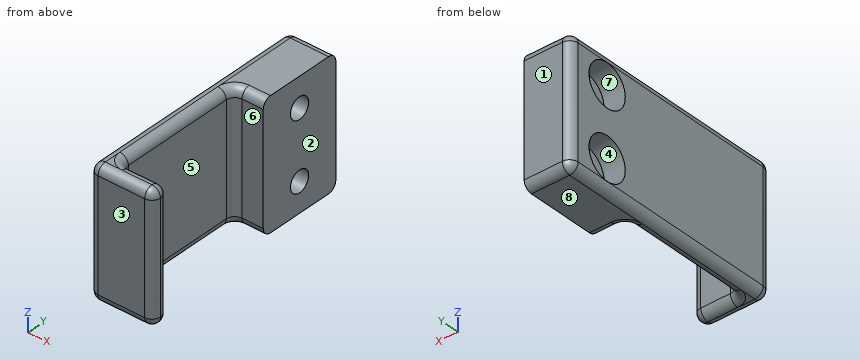
```python
from build123d import *

# Parameters (mm, degrees)
EXTRUDE_1_DEPTH     = 30
SKETCH_3_W          = 7
SKETCH_3_H          = 20
EXTRUDE_2_DEPTH     = 30
SKETCH_2_R          = 2.5
CUT_EXTRUDE_1_DEPTH = 30
FILLET_1_R          = 2
FILLET_2_R          = 2
FILLET_3_R          = 2
FILLET_5_R          = 2
SKETCH_4_R          = 5
CUT_EXTRUDE_2_DEPTH = 5


with BuildPart() as part:
    # 스케치1 → 보스-돌출1 (new body)
    with BuildSketch(Plane.XY):
        Polygon((-41.818181818, 31.136363636), (-37.818181818, 31.136363636), (-37.818181818, -19.863636364), (-26.818181818, -19.863636364), (-26.818181818, -23.863636364), (-32.727272727, -23.863636364), (-41.818181818, -23.863636364), align=None)
    extrude(amount=EXTRUDE_1_DEPTH)

    # 스케치3 → 보스-돌출2 (add)
    with BuildSketch(Plane.XY.offset(30)):
        with Locations((-34.318181818, 21.136363636)):
            Rectangle(SKETCH_3_W, SKETCH_3_H)
    extrude(amount=-EXTRUDE_2_DEPTH)

    # 스케치2 → 컷-돌출1 (cut)
    with BuildSketch(Plane.ZY.offset(41.818181818)):
        with Locations((7, 21.136363636)):
            Circle(SKETCH_2_R)
        with Locations((23, 21.136363636)):
            Circle(SKETCH_2_R)
    extrude(amount=-CUT_EXTRUDE_1_DEPTH, mode=Mode.SUBTRACT)

    # 필렛1
    fillet_1_edges = [part.edges().sort_by_distance(p)[0] for p in [
        (-37.818181818, -19.863636364, 15),
        (-37.818181818, 11.136363636, 15),
    ]]
    fillet(fillet_1_edges, radius=FILLET_1_R)

    # 필렛2
    fillet_2_edges = [part.edges().sort_by_distance(p)[0] for p in [
        (-41.818181818, -23.863636364, 15),
    ]]
    fillet(fillet_2_edges, radius=FILLET_2_R)

    # 필렛3
    fillet_3_edges = [part.edges().sort_by_distance(p)[0] for p in [
        (-26.818181818, -23.863636364, 15),
        (-26.818181818, -19.863636364, 15),
        (-41.818181818, 31.136363636, 15),
    ]]
    fillet(fillet_3_edges, radius=FILLET_3_R - 0.0001)  # a hair under: the kernel refuses the full size

    # 필렛5
    fillet_5_edges = [part.edges().sort_by_distance(p)[0] for p in [
        (-35.318231818, 31.136363636, 30),
        (-33.318181818, 11.136363636, 0),
        (-37.818181818, -4.363636364, 0),
        (-37.818181818, -4.363636364, 30),
        (-33.318181818, 11.136363636, 30),
        (-37.232395381, 10.550577199, 30),
        (-37.232395381, 10.550577199, 0),
        (-37.232395381, -19.277849926, 0),
        (-37.232395381, -19.277849926, 30),
        (-34.318131818, -23.863636364, 0),
        (-34.318131818, -23.863636364, 30),
        (-41.232395381, -23.277849926, 0),
        (-41.232395381, -23.277849926, 30),
        (-41.818181818, 3.636413636, 0),
        (-32.318131818, -19.863636364, 0),
        (-41.23242467, 30.550606488, 0),
        (-27.403938966, -20.449393512, 0),
        (-27.403938966, -23.277879215, 0),
        (-41.818181818, 3.636413636, 30),
        (-35.318231818, 31.136363636, 0),
        (-32.318131818, -19.863636364, 30),
        (-41.23242467, 30.550606488, 30),
        (-27.403938966, -20.449393512, 30),
        (-27.403938966, -23.277879215, 30),
    ]]
    fillet(fillet_5_edges, radius=FILLET_5_R - 0.0001)  # a hair under: the kernel refuses the full size

    # 스케치4 → 컷-돌출2 (cut)
    with BuildSketch(Plane.ZY.offset(41.818181818)):
        with Locations((7, 21.136363636)):
            Circle(SKETCH_4_R)
        with Locations((23, 21.136363636)):
            Circle(SKETCH_4_R)
    extrude(amount=-CUT_EXTRUDE_2_DEPTH, mode=Mode.SUBTRACT)


solid = part.part
```
Geometry check sheet. Reference: the model listing, model coordinates, mm. Face numbers are marked on the shaded views. A direction names the side the tool comes from. Coordinates: 2 decimals unless noted, no trailing zeros.
Item 1: Section check B-B (x = -34). Count the separate pieces of the cut face and the enclosed holes in it, plus the area to 3 significant figures.
Item 2: Scan lines: line 1 along Y through (x, z) = (-34.9, 23); line 2 along Y through (x, z) = (-33, 22.25); line 3 along Y through (x, z) = (-35.75, 27.5). Record each from-to range of solid material in increasing order.
Item 3: Tool access check on the marked faces 1, 2, 3, 4 and 5. Record the directions out of +Z, -Z, +X, -X, +Y, -Y that give a thin tool (end or side, any length) a straight path to the whole face; none if there is none.
Item 4: Depth check by flat-ended pin: pin 1 (5 mm diameter, centred on y = 23, z = 5.5, fed in from -X); pin 2 (8 mm diameter, centred on y = -7.5, z = 12, fed in from +X); pin 3 (9 mm diameter, centred on y = 21.14, z = 23, fed in from +X); pin 4 (4.5 mm diameter, centred on y = 21.14, z = 7, fed in from -X). Enter the tip coordinate at first touch or a pass-through.
Item 5: Mould release check, pull along Z, two halves, no side actions. Record for the marked faces 6, 7 and 8: released by +Z, released by -Z, zero draft, split by the parting line, or undercut.
Check sheet entries:
1. separate pieces: 2
1. enclosed holes: 2
1. area: 674 mm2
2. line 1: y = -23.86 to -19.86, 11.14 to 18.64, 23.64 to 31.14
2. line 2: y = -23.86 to -19.86, 11.14 to 18.75, 23.52 to 31.14
2. line 3: y = -23.86 to -19.86, 11.14 to 31.14
3. face 1: +Z, -Z, +X, -X, +Y
3. face 2: +Z, -Z, +X, +Y
3. face 3: +Z, -Z, +X, -X, -Y
3. face 4: -X
3. face 5: +Z, -Z, +X
4. pin 1: stops at x = -36.82
4. pin 2: stops at x = -37.82
4. pin 3: stops at x = -30.82
4. pin 4: passes through
5. face 6: zero draft
5. face 7: undercut
5. face 8: released by -Z
